```python
from build123d import *

# Parameters (mm, degrees)
SKETCH1_R           = 750
SKETCH1_R_2         = 8.89
BOSS_EXTRUDE1_DEPTH = 20
FILLET1_R           = 10
SKETCH3_R           = 5
BOSS_EXTRUDE2_DEPTH = 47


with BuildPart() as part:
    # Sketch1 → Boss-Extrude1 (new body)
    with BuildSketch(Plane(origin=(0, 0, 0), x_dir=(1, 0, 0), z_dir=(0, 1, 0))):
        with Locations(Location((0, 0, 0), (0, 0, 270))):
            Circle(SKETCH1_R)
        with Locations(Location((0, 300, 0), (0, 0, 270))):
            Circle(SKETCH1_R_2, mode=Mode.SUBTRACT)
        with Locations(Location((-300, 0, 0), (0, 0, 270))):
            Circle(SKETCH1_R_2, mode=Mode.SUBTRACT)
        with Locations(Location((300, 0, 0), (0, 0, 270))):
            Circle(SKETCH1_R_2, mode=Mode.SUBTRACT)
    extrude(amount=BOSS_EXTRUDE1_DEPTH)

    # Fillet1
    fillet1_edges = [part.edges().sort_by_distance(p)[0] for p in [
        (0, 0, -750),
        (-300, 0, -8.89),
        (300, 0, -8.89),
        (0, 0, -308.89),
    ]]
    fillet(fillet1_edges, radius=FILLET1_R)

    # Sketch3 → Boss-Extrude2 (add)
    with BuildSketch(Plane(origin=(0, 20, 0), x_dir=(1, 0, 0), z_dir=(0, 1, 0))):
        with Locations(Location((-325, 0, 0), (0, 0, 270))):
            Circle(SKETCH3_R)
        with Locations(Location((325, 0, 0), (0, 0, 270))):
            Circle(SKETCH3_R)
        with Locations(Location((0, 325, 0), (0, 0, 270))):
            Circle(SKETCH3_R)
    extrude(amount=-BOSS_EXTRUDE2_DEPTH)


solid = part.part
```
Check sheet for the modelled part. Datum: model origin and axes. Units: mm. Coordinates: 2 decimals unless noted, no trailing zeros. Loops run counter-clockwise (first coordinate to the right, second up) from the corner with the lowest first, then second, coordinate; pieces in that order, holes last. Notation, with made-up numbers: M 84.25,58 L 133.25,58 A15 ccw 133.25,70 Z; hole C 74.25,23.25 d9. An arc over 180 degrees is marked long. Answer as a JSON object with one key per item and string values.
1. Sectioned sample at A-A on y = -10.5. Record the cut outline in (x, z).
Outcome:
{"outline": "C -325,0 d10; C 0,-325 d10; C 325,0 d10"}
2. Depth check by flat-ended pin: P1, Ø5, axis at x = -242.5, z = 115.5, coming from the -Y side; P2, Ø3, axis at y = 9, z = 358, coming from the +X side; P3, Ø23, axis at x = 0, z = -300, coming from the -Y side; P4, Ø16, axis at x = 300, z = 0, coming from the +Y side. Enter the tip coordinate at first touch or a pass-through.
Outcome:
{"P1": "y = 0", "P2": "x = 659.81", "P3": "y = 3.26", "P4": "through"}
3. Scan lines: L1, parallel to X at y = 16, z = 0; L2, parallel to Y at x = -135.5, z = -234; L3, parallel to Z at x = 323, y = -16. Record each from-to range of solid material in increasing order. Write a range as from..to.
Outcome:
{"L1": "-750..-308.89, -291.11..291.11, 308.89..750", "L2": "0..20", "L3": "-4.58..4.58"}
